Geometry check sheet. Reference: the model listing, model coordinates, mm. Give positions to 0.01 mm unless a question says otherwise; leave off trailing zeros. Loops run counter-clockwise (first coordinate to the right, second up) from the corner with the lowest first, then second, coordinate; pieces in that order, holes last.
1. Go/stop test with flat-tipped pins: pin 1 Ø3.5 at (x, z) = (-70.5, 0.5) entering from -Y; pin 2 Ø3 at (y, z) = (6, 4.5) entering from -X; pin 3 Ø3.5 at (y, z) = (65.5, 0) entering from +X. Record where each tip stops, or that it passes through.
2. Cross-section at A-A, the plane y = 34.5. Record the cut outline in (x, z).
3. Material ranges on L1, parallel to Y at x = -251, z = 3; L2, parallel to Y at x = 50.5, z = 2.25; L3, parallel to X at y = 34.5, z = 3.75, recorded low to high.
4. Cross-section at C-C, the plane x = -149.5. Record the cut outline in (y, z).
5. Cross-section at B-B, the plane z = -1.5. Record the cut outline in (x, y).
Autodesk Inventor part; units mm, degrees
ref_plane "Work Plane1" through (250, 69, 0) normal (-1, 0, 0) x (0, -1, 0)
ref_plane "YZ Plane" through (0, 0, 0) normal (1, 0, 0) x (0, 1, 0)
ref_plane "XZ Plane" through (0, 0, 0) normal (0, 1, 0) x (-1, 0, 0)
sketch "Sketch1" plane through (0, 0, 0) normal (0, 0, 1) x (1, 0, 0)
  line L0 (250, 69) -> (-250, 69)
  line L1 (-53.0332, 0) -> (53.0332, 0) construction
  arc A0 (-250, 69) -> (-250, 0) centre (-250, 34.5) ccw
  line L2 (-250, 0) -> (-240, 0)
  point P0 (0, 0)
  point P1 (0, 69)
  point P2 (0, 0)
  dimension "d0" = 500
  dimension "d1" = 69
  dimension "d25" = 10
ref_plane "Work Plane1" through (250, 69, 0) normal (-1, 0, 0) x (0, -1, 0)
sketch "Sketch2" plane through (250, 69, 0) normal (-1, 0, 0) x (0, -1, 0)
  line L0 (3.5, 3.5) -> (-3.5, 3.5)
  line L1 (-3.5, 3.5) -> (-3.5, -3.5)
  line L2 (-3.5, -3.5) -> (3.5, -3.5)
  line L3 (3.5, -3.5) -> (3.5, 3.5)
  line L4 (-5.5, 5.5) -> (5.5, 5.5)
  line L5 (5.5, 5.5) -> (5.5, -5.5)
  line L6 (5.5, -5.5) -> (-5.5, -5.5)
  line L7 (-5.5, -5.5) -> (-5.5, 5.5)
  point P0 (69, 0)
  point P1 (0, 3.5)
  point P2 (3.5, 0)
  point P3 (0, 0)
  point P4 (0, 0)
  point P5 (0, 0)
  dimension "d2" = 7
  dimension "d3" = 7
  dimension "d4" = 2
sweep "Sweep1" add profiles "Sketch2" path "Sketch1"
sketch "Sketch3" plane through (250, 63.5, 5.5) normal (0, 0, 1) x (1, 0, 0)
  line L0 (0, 9) -> (-500, 9)
  line L1 (0, 9) -> (-10, 7.2367)
  line L2 (-10, 7.2367) -> (-10, 0)
  line L3 (0, 0) -> (-500, 0)
  line L4 (0, 0) -> (-500, 0)
  line L5 (0, 0) -> (0, 11)
  line L6 (-500, -67) -> (-490, -67)
  line L7 (-490, -67) -> (-500, -65.2367)
  line L8 (-500, -65.2367) -> (-500, -58)
  line L9 (-490, -58) -> (-490, -69)
  line L10 (-500, -58) -> (-490, -58)
  dimension "d29" = 100
  dimension "d30" = 10
  dimension "d33" = 100
  dimension "d34" = 10
extrude "Extrusion1" cut sketch "Sketch3" against normal through all
properties part number "0008-10-1026 wire chain Y"
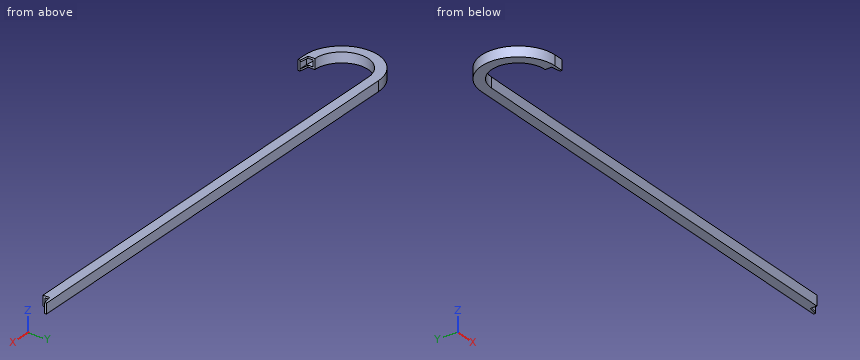
Result:
1. pin 1: stops at y = 63.5
1. pin 2: stops at x = -279.51
1. pin 3: stops at x = 240
2. outline: (-290, -5.5) - (-279, -5.5) - (-279, 5.5) - (-290, 5.5) - close; hole (-288, -3.5) - (-281, -3.5) - (-281, 3.5) - (-288, 3.5) - close
3. L1: y = -5.49 to -3.49, 3.52 to 5.52, 63.48 to 65.48, 72.49 to 74.49
3. L2: y = 63.5 to 65.5, 72.5 to 74.5
3. L3: x = -290 to -279
4. outline: (63.5, -5.5) - (74.5, -5.5) - (74.5, 5.5) - (63.5, 5.5) - close; hole (65.5, -3.5) - (72.5, -3.5) - (72.5, 3.5) - (65.5, 3.5) - close
5. outline: (-250, -5.5) - (-240, -5.5) - (-240, -3.5) - (-250, -3.5) arc R38 cw to (-250, 72.5) - (250, 72.5) - (250, 74.5) - (-250, 74.5) arc R40 ccw to start; (-250, 3.5) - (-250, 5.5) arc R29 cw to (-250, 63.5) - (240, 63.5) - (240, 65.5) - (-250, 65.5) arc R31 ccw to start
